The listing builds one solid part. Answer for the finished solid, in the listing's coordinates (mm). Face numbers are marked on the shaded views. A direction names the side the tool comes from. Round coordinates to 2 decimals unless told otherwise and drop trailing zeros. Write each loop counter-clockwise with the first axis right and the second up, starting at its lowest first coordinate (ties: lowest second). Pieces come first, ordered by that corner, then holes. Notation, with made-up numbers: (70.5, 27) - (111.5, 27) arc R17 cw to (111.5, 60) - close; hole circle Ø10 at (-2.5, 36.5). An arc over 180 degrees is marked (long way). Return JSON: item names as keys, results as strings. Group by question number.
(1) Each of these flat-tipped pins is pushed along its axis until it touches: pin 1 (2 mm diameter, centred on x = 121, z = -2, fed in from -Y); pin 2 (1 mm diameter, centred on x = 92.5, z = -5.5, fed in from +Y); pin 3 (2 mm diameter, centred on x = 120, z = -2, fed in from +Y). Where does it stop, or does it pass through?
(2) Section C-C, the plane y = -14 is taken. Write down the section's boundary in (x, z).
(3) Which of the six approach directions +Z, -Z, +X, -X, +Y, -Y give full straight-line access (tool end or side, diameter ignored) to the marked faces 1 and 2?
(4) Section B-B, the plane x = 142 is taken. Write down the section's boundary in (y, z), then the cut area to 3 significant figures.
(5) Find the intervals of material crossed by line 1 along X through (y, z) = (-2.3, -17); line 2 along Y through (x, z) = (126, -21.5); line 3 along Z through (x, y) = (49.5, -23.5), in increasing order. Write a range as [from, to].
(6) Section D-D, the plane x = 8 is taken. Write down the section's boundary in (y, z).
(7) Section A-A, the plane z = -17 is taken. Write down the section's boundary in (x, y), then the cut area to 3 significant figures.
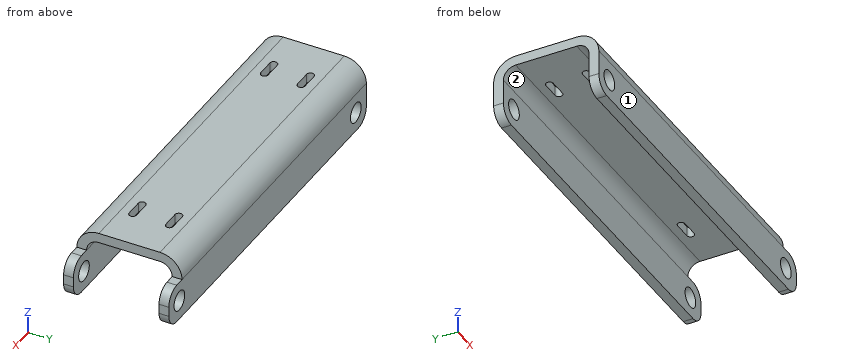
```python
from build123d import *

# Parameters (mm, degrees)
EXTRUSION_DEPTH  = 150
SKETCH_4_R       = 4.05
HOLES_DEPTH      = 159.031642401
SKETCH_5_W       = 10
SKETCH_5_H       = 9
SLOT_DEPTH       = 159.031642401
FILLET_2_R       = 6
MORE_HOLES_DEPTH = 4


# Sheet-metal steps are written as plain solids
with BuildPart() as part:
    # Sketch 1 → Extrusion (new body)
    with BuildSketch(Plane(origin=(0, 0, 0), x_dir=(0, 0, -1), z_dir=(1, 0, 0))):
        with BuildLine():
            Line((25, -43), (9, -43))
            ThreePointArc((9, -43), (2.636038969, -40.363961031), (0, -34))
            Line((0, -34), (0, -9))
            ThreePointArc((0, -9), (2.636038969, -2.636038969), (9, 0))
            Line((9, 0), (25, 0))
            Line((25, 0), (25, -4))
            Line((25, -4), (9, -4))
            ThreePointArc((9, -4), (5.464466094, -5.464466094), (4, -9))
            Line((4, -9), (4, -34))
            ThreePointArc((4, -34), (5.464466094, -37.535533906), (9, -39))
            Line((9, -39), (25, -39))
            Line((25, -39), (25, -43))
        make_face()
    extrude(amount=EXTRUSION_DEPTH)

    # Эскиз4 → Holes (cut, through all)
    with BuildSketch(Plane(origin=(0, 0, 0), x_dir=(1, 0, 0), z_dir=(0, 1, 0))):
        with Locations(Location((8, 17, 0), (0, 0, 270))):
            Circle(SKETCH_4_R)
        with Locations(Location((142, 17, 0), (0, 0, 270))):
            Circle(SKETCH_4_R)
    extrude(amount=-HOLES_DEPTH, mode=Mode.SUBTRACT)

    # Эскиз5 → SLot (cut, through all)
    with BuildSketch(Plane.XZ.offset(43)):
        with Locations((145, -4.5)):
            Rectangle(SKETCH_5_W, SKETCH_5_H)
    extrude(amount=-SLOT_DEPTH, mode=Mode.SUBTRACT)

    # Fillet 2
    fillet_2_edges = [part.edges().sort_by_distance(p)[0] for p in [
        (0, -41, -25),
        (0, -2, -25),
        (150, -41, -25),
        (150, -2, -9),
        (150, -41, -9),
        (150, -2, -25),
    ]]
    fillet(fillet_2_edges, radius=FILLET_2_R)

    # Эскиз6 → More Holes (cut)
    with BuildSketch(Plane.XY):
        with BuildLine():
            Line((16.5, -12.5), (23.5, -12.5))
            ThreePointArc((23.5, -12.5), (25, -14), (23.5, -15.5))
            Line((23.5, -15.5), (16.5, -15.5))
            ThreePointArc((16.5, -15.5), (15, -14), (16.5, -12.5))
        make_face()
        with BuildLine():
            Line((123.5, -12.5), (116.5, -12.5))
            ThreePointArc((116.5, -12.5), (115, -14), (116.5, -15.5))
            Line((116.5, -15.5), (123.5, -15.5))
            ThreePointArc((123.5, -15.5), (125, -14), (123.5, -12.5))
        make_face()
        with BuildLine():
            Line((123.5, -30.5), (116.5, -30.5))
            ThreePointArc((116.5, -30.5), (115, -29), (116.5, -27.5))
            Line((116.5, -27.5), (123.5, -27.5))
            ThreePointArc((123.5, -27.5), (125, -29), (123.5, -30.5))
        make_face()
        with BuildLine():
            Line((16.5, -30.5), (23.5, -30.5))
            ThreePointArc((23.5, -30.5), (25, -29), (23.5, -27.5))
            Line((23.5, -27.5), (16.5, -27.5))
            ThreePointArc((16.5, -27.5), (15, -29), (16.5, -30.5))
        make_face()
    extrude(amount=-MORE_HOLES_DEPTH, mode=Mode.SUBTRACT)


solid = part.part
```
Working result:
{
 "1": {"pin 1": "stops at y = -40.71", "pin 2": "stops at y = -0.51", "pin 3": "stops at y = -2.29"},
 "2": {"outline": "(0, -4) - (15, -4) - (15, 0) - (0, 0) - close; (25, -4) - (115, -4) - (115, 0) - (25, 0) - close; (125, -4) - (140, -4) - (140, 0) - (125, 0) - close"},
 "3": {"face 1": "+Z, -Z, +X, -X, -Y", "face 2": "-Z, +X, -X"},
 "4": {"outline": "(-43, -25) - (-39, -25) - (-39, -21.05) - (-43, -21.05) - close; (-43, -12.95) - (-39, -12.95) - (-39, -9) - (-43, -9) - close; (-4, -25) - (0, -25) - (0, -21.05) - (-4, -21.05) - close; (-4, -12.95) - (0, -12.95) - (0, -9) - (-4, -9) - close", "area": "63.2 mm^2"},
 "5": {"line 1": "x = [0, 3.95], [12.05, 137.95], [146.05, 150]", "line 2": "y = [-43, -39], [-4, 0]", "line 3": "z = [-4, 0]"},
 "6": {"outline": "(-43, -25) - (-39, -25) - (-39, -21.05) - (-43, -21.05) - close; (-43, -12.95) - (-39, -12.95) - (-39, -9) arc R5 cw to (-34, -4) - (-9, -4) arc R5 cw to (-4, -9) - (-4, -12.95) - (0, -12.95) - (0, -9) arc R9 ccw to (-9, 0) - (-34, 0) arc R9 ccw to (-43, -9) - close; (-4, -25) - (0, -25) - (0, -21.05) - (-4, -21.05) - close"},
 "7": {"outline": "(0, -43) - (3.95, -43) - (3.95, -39) - (0, -39) - close; (0, -4) - (3.95, -4) - (3.95, 0) - (0, 0) - close; (12.05, -43) - (137.95, -43) - (137.95, -39) - (12.05, -39) - close; (12.05, -4) - (137.95, -4) - (137.95, 0) - (12.05, 0) - close; (146.05, -43) - (150, -43) - (150, -39) - (146.05, -39) - close; (146.05, -4) - (150, -4) - (150, 0) - (146.05, 0) - close", "area": "1,070 mm^2"}
}
